Work out the finished part from the listing and answer in its coordinate system (mm). A direction names the side the tool comes from. Round coordinates to 2 decimals unless told otherwise and drop trailing zeros. Order: outer loops, then holes, each group sorted by start corner. A loop starts at its lowest first (then second) coordinate and runs counter-clockwise, first axis right, second up. Notation, with made-up numbers: (38.5, -14.5) -> (51.5, -14.5) arc R10 cw to (51.5, 4.5) -> close; hole circle Ø4 at (19.5, -21). An arc over 180 degrees is marked (long way). Use one line per item in the form item = value.
Autodesk Inventor part; units mm, degrees
ref_plane "YZ Plane" through (0, 0, 0) normal (1, 0, 0) x (0, 1, 0)
ref_plane "XZ Plane" through (0, 0, 0) normal (0, 1, 0) x (-1, 0, 0)
ref_plane "XY Plane" through (0, 0, 0) normal (0, 0, 1) x (1, 0, 0)
sketch "スケッチ4" plane through (0, 0, 0) normal (0, 0, 1) x (1, 0, 0)
  circle A0 centre (-7.8, 0) radius 7.8
  circle A1 centre (7.8, 0) radius 7.8
  line L0 (-15.6, -7.8) -> (15.6, -7.8)
  line L1 (15.6, -7.8) -> (15.6, 7.8)
  line L2 (15.6, 7.8) -> (-15.6, 7.8)
  line L3 (-15.6, 7.8) -> (-15.6, -7.8)
  line L4 (-16.6, 8.8) -> (16.6, 8.8)
  line L5 (16.6, 8.8) -> (16.6, -8.8)
  line L6 (16.6, -8.8) -> (-16.6, -8.8)
  line L7 (-16.6, -8.8) -> (-16.6, 8.8)
  line L8 (-1.8133, 5) -> (1.8133, 5)
  line L9 (-1.8133, -5) -> (1.8133, -5)
  point P0 (0, 0)
  dimension "d12" = 15.6
  dimension "d13" = 1
  dimension "d14" = 10
extrude "押し出し4" add sketch "スケッチ4" along normal blind 10 contours A0 L2 A1 L8 | L9 A1 L0 A0 | A0 L3 L2 | L0 L3 A0 | L2 L1 A1 | A1 L1 L0 | L4 L5 L6 L7
sketch "スケッチ5" plane through (0, 0, 0) normal (0, 0, -1) x (-1, 0, 0)
  arc A0 (-1.8133, 5) -> (-1.8133, -5) centre (-7.8, 0) ccw
  line L0 (-1.8133, 5) -> (1.8133, 5)
  arc A1 (1.8133, -5) -> (1.8133, 5) centre (7.8, 0) ccw
  line L1 (1.8133, -5) -> (-1.8133, -5)
  line L2 (16.6, 8.8) -> (-16.6, 8.8)
  line L3 (-16.6, 8.8) -> (-16.6, -8.8)
  line L4 (-16.6, -8.8) -> (16.6, -8.8)
  line L5 (16.6, -8.8) -> (16.6, 8.8)
  point P0 (0, 0)
extrude "押し出し5" add sketch "スケッチ5" along normal blind 1.5 contours L0 A1 L1 A0 | L5 L4 L3 L2
sketch "スケッチ6" plane through (-16.6, 8.8, 10) normal (0, 1, 0) x (1, 0, 0)
  line L0 (14.7867, 10) -> (14.7867, 10) construction
  line L1 (14.7867, 10) -> (14.7867, 0) construction
  line L2 (14.7867, 0) -> (14.7867, 0) construction
  line L3 (14.7867, 10) -> (14.7867, 0) construction
  line L4 (18.4133, 10) -> (18.4133, 10) construction
  line L5 (18.4133, 10) -> (18.4133, 0) construction
  line L6 (18.4133, 0) -> (18.4133, 0) construction
  line L7 (18.4133, 10) -> (18.4133, 0) construction
  line L8 (18.4133, 10) -> (18.4133, 10) construction
  line L9 (18.4133, 10) -> (14.7867, 10) construction
  line L10 (14.7867, 10) -> (14.7867, 10) construction
  line L11 (14.7867, 10) -> (18.4133, 10) construction
  line L12 (14.7867, 10) -> (1, 10) construction
  line L13 (1, 10) -> (1, 8) construction
  line L14 (1, 8) -> (16.6, 8) construction
  line L15 (14.7867, 8) -> (14.7867, 10) construction
  line L16 (32.2, 10) -> (32.2, 0) construction
  line L17 (18.4133, 10) -> (32.2, 10) construction
  line L18 (32.2, 10) -> (32.2, 8) construction
  line L19 (32.2, 8) -> (16.6, 8) construction
  line L20 (18.4133, 7.5) -> (18.4133, 10) construction
  line L21 (4.05, 10) -> (13.55, 10)
  line L22 (13.55, 10) -> (13.55, 8)
  line L23 (13.55, 8) -> (4.05, 8)
  line L24 (4.05, 8) -> (4.05, 10)
  line L25 (18.4133, 10) -> (32.2, 10)
  line L26 (19.65, 10) -> (29.15, 10)
  line L27 (29.15, 10) -> (29.15, 8)
  line L28 (29.15, 8) -> (19.65, 8)
  line L29 (19.65, 8) -> (19.65, 10)
  line L30 (1, 10) -> (16.6, 10)
  line L31 (16.6, 10) -> (16.6, 7)
  line L32 (16.6, 7) -> (1, 7)
  line L33 (1, 7) -> (1, 10)
  line L34 (32.2, 10) -> (16.6, 10)
  line L35 (16.6, 10) -> (16.6, 7)
  line L36 (16.6, 7) -> (32.2, 7)
  line L37 (32.2, 7) -> (32.2, 10)
  line L38 (6.05, 8) -> (11.55, 8)
  line L39 (11.55, 8) -> (11.55, 7)
  line L40 (11.55, 7) -> (6.05, 7)
  line L41 (6.05, 7) -> (6.05, 8)
  line L42 (21.65, 8) -> (27.15, 8)
  line L43 (27.15, 8) -> (27.15, 7)
  line L44 (27.15, 7) -> (21.65, 7)
  line L45 (21.65, 7) -> (21.65, 8)
  point P0 (16.6, 10)
  point P1 (24.4, 8)
  point P2 (8.8, 8)
  dimension "d19" = 2
  dimension "d20" = 9.5
  dimension "d21" = 1
  dimension "d22" = 5.5
extrude "押し出し6" cut sketch "スケッチ6" against normal blind 15 contours L21 L22 L23 L24 | L23 L39 L32 L41 | L45 L28 L43 L36 | L25 L27 L28 L29
extrude "押し出し7" add sketch "スケッチ6" against normal blind 16 contours L24 L23 L41 L32 L33 L30 | L30 L31 L32 L39 L23 L22 | L34 L25 L29 L28 L45 L36 L31 | L43 L28 L27 L25 L37 L36
sketch "スケッチ7" plane through (0, 0, -1.5) normal (0, 0, -1) x (-1, 0, 0)
  line L0 (12.55, 8.8) -> (12.55, -6.2) construction
  line L1 (3.05, 8.8) -> (3.05, -6.2) construction
  line L2 (12.55, 8.8) -> (3.05, 8.8) construction
  line L3 (-12.55, 8.8) -> (-12.55, -6.2) construction
  line L4 (-3.05, 8.8) -> (-12.55, 8.8) construction
  line L5 (-3.05, 8.8) -> (-3.05, -6.2) construction
  line L6 (-3.05, 8.8) -> (-3.05, -6.2)
  line L7 (-12.55, 8.8) -> (-3.05, 8.8)
  line L8 (-3.05, 8.8) -> (-3.05, 5.8)
  line L9 (-3.05, 5.8) -> (-12.55, 5.8)
  line L10 (-12.55, 5.8) -> (-12.55, 8.8)
  line L11 (3.05, 8.8) -> (12.55, 8.8)
  line L12 (12.55, 8.8) -> (12.55, 5.8)
  line L13 (12.55, 5.8) -> (3.05, 5.8)
  line L14 (3.05, 5.8) -> (3.05, 8.8)
  line L15 (-3.05, -6.2) -> (-3.0671, -6.2)
  arc A0 (-12.5329, -6.2) -> (-3.0671, -6.2) centre (-7.8, 0) ccw
  line L16 (-12.5329, -6.2) -> (-12.55, -6.2)
  line L17 (12.55, -6.2) -> (12.5329, -6.2)
  arc A1 (3.0671, -6.2) -> (12.5329, -6.2) centre (7.8, 0) ccw
  line L18 (3.0671, -6.2) -> (3.05, -6.2)
  point P0 (0, 0)
  point P1 (-3.05, -5.2)
  dimension "d27" = 3
extrude "押し出し8" cut sketch "スケッチ7" against normal up to next
fillet "フィレット1" radius 8 4 edges at (16.6, 8.8, 4.25) (16.6, -8.8, 4.25) (-16.6, 8.8, 4.25) (-16.6, -8.8, 4.25)
properties part number "CaseBottom_CR123A"
Item 1: Flat-ended cylindrical pins translate along their axes: P1, Ø0.8, axis at y = 4.5, z = 2.5, coming from the -X side; P2, Ø0.8, axis at x = 8, z = -1, coming from the +Y side; P3, Ø1, axis at y = 4, z = -0.5, coming from the +X side. Find the tip coordinate at first contact, or state that the pin passes through.
Findings:
P1 = -15.89
P2 = 5.8
P3 = 16.13
Item 2: Determine the mould class of faces 1 (the flat face through (-0.1, -5.2, 10)), 2 (the flat face through (8, 8, 3)), 3 (the cylindrical face through (14.194, 6.519, 4.17)) for opening direction X: released by +X, released by -X, zero draft, split by the parting line, or undercut.
Findings:
face_1 = zero draft
face_2 = undercut
face_3 = released by +X
Item 3: The part is cut by section D-D, the plane z = 8.5. Give the vertices of the cut face in (x, y), and give its area (3 significant figures).
Findings:
outline = (-16.6, -0.8) arc R8 ccw to (-8.6, -8.8) -> (8.6, -8.8) arc R8 ccw to (16.6, -0.8) -> (16.6, 0.8) arc R8 ccw to (8.6, 8.8) -> (-8.6, 8.8) arc R8 ccw to (-16.6, 0.8) -> close; hole (-1.81, -5) -> (1.81, -5) arc R7.8 ccw (long way) to (1.81, 5) -> (-1.81, 5) arc R7.8 ccw (long way) to start
area = 136 mm^2
Item 4: The part is cut by section B-B, the plane x = 7.8. Give the vertices of the cut face in (y, z), and give its area (3 significant figures).
Findings:
outline = (-8.8, -1.5) -> (5.8, -1.5) -> (5.8, 0) -> (-7.8, 0) -> (-7.8, 10) -> (-8.8, 10) -> close; (7.8, 3) -> (8.8, 3) -> (8.8, 10) -> (7.8, 10) -> close
area = 38.9 mm^2
Item 5: The part is cut by section C-C, the plane y = 0. Give the vertices of the cut face in (x, z).
Findings:
outline = (-16.6, -1.5) -> (16.6, -1.5) -> (16.6, 10) -> (15.6, 10) -> (15.6, 3) -> (10.55, 3) -> (10.55, 2) -> (12.55, 2) -> (12.55, 0) -> (3.05, 0) -> (3.05, 2) -> (5.05, 2) -> (5.05, 3) -> (-5.05, 3) -> (-5.05, 2) -> (-3.05, 2) -> (-3.05, 0) -> (-12.55, 0) -> (-12.55, 2) -> (-10.55, 2) -> (-10.55, 3) -> (-15.6, 3) -> (-15.6, 10) -> (-16.6, 10) -> close
Item 6: For faces 4 (the flat face through (0, -5, 6)), 5 (the flat face through (-16.6, 0, 4)), 6 (the flat face through (0, -2, -1.5)), 7 (the flat face through (-8, 5.8, -1)), 8 (the flat face through (-12, 1, 2)), determine the directions among +Z, -Z, +X, -X, +Y, -Y from which every point of the face is accessible in a straight line to the end or side of a thin tool.
Findings:
face_4 = +Z
face_5 = +Z, -Z, -X, +Y, -Y
face_6 = -Z, +X, -X, +Y, -Y
face_7 = -Z, +Y
face_8 = +Y
Item 7: Consider line 1 along X through (y, z) = (0, 7); line 2 along Y through (x, z) = (7.8, 8.25); line 3 along Y through (x, z) = (0, 5.75). Determine where each line is inside the solid, lowest interval first.
Findings:
line_1 = -16.6 to -15.6, 15.6 to 16.6
line_2 = -8.8 to -7.8, 7.8 to 8.8
line_3 = -8.8 to -5, 5 to 8.8
Item 8: The part is cut by section A-A, the plane y = 6.5. Give the vertices of the cut face in (x, z), and give its area (3 significant figures).
Findings:
outline = (-14.21, -1.5) -> (-12.55, -1.5) -> (-12.55, 2) -> (-10.55, 2) -> (-10.55, 3) -> (-12.11, 3) -> (-12.11, 10) -> (-14.21, 10) -> close; (-5.05, 2) -> (-3.05, 2) -> (-3.05, -1.5) -> (3.05, -1.5) -> (3.05, 2) -> (5.05, 2) -> (5.05, 3) -> (3.49, 3) -> (3.49, 10) -> (-3.49, 10) -> (-3.49, 3) -> (-5.05, 3) -> close; (10.55, 2) -> (12.55, 2) -> (12.55, -1.5) -> (14.21, -1.5) -> (14.21, 10) -> (12.11, 10) -> (12.11, 3) -> (10.55, 3) -> close
area = 129 mm^2
